Autodesk Inventor part; units mm, degrees
ref_plane "YZ Plane" through (0, 0, 0) normal (1, 0, 0) x (0, 1, 0)
ref_plane "XZ Plane" through (0, 0, 0) normal (0, 1, 0) x (-1, 0, 0)
ref_plane "XY Plane" through (0, 0, 0) normal (0, 0, 1) x (1, 0, 0)
sketch "Skizze1" plane through (0, 0, 0) normal (0, 0, 1) x (1, 0, 0)
  line L0 (-2.05, 0.55) -> (2.05, 0.55)
  line L1 (2.05, 0.55) -> (2.05, -0.55)
  line L2 (2.05, -0.55) -> (-2.05, -0.55)
  line L3 (-2.05, -0.55) -> (-2.05, 0.55)
  line L4 (-0.65, 2.05) -> (0.65, 2.05)
  line L5 (0.65, 2.05) -> (0.65, -2.05)
  line L6 (0.65, -2.05) -> (-0.65, -2.05)
  line L7 (-0.65, -2.05) -> (-0.65, 2.05)
  circle A0 centre (0, 0) radius 3.5
  line L8 (-4.9, 0) -> (4.9, 0) construction
  line L9 (0, -4.9) -> (0, 4.9) construction
  point P0 (0.65, -0.55)
  point P1 (-0.65, -0.55)
  point P2 (-0.65, 0.55)
  point P3 (0.65, 0.55)
  dimension "d0" = 1.3
  dimension "d1" = 1.1
  dimension "d2" = 4.1
  dimension "d3" = 4.1
  dimension "d4" = 7
extrude "Extrusion1" add sketch "Skizze1" along normal blind 5
sketch "Skizze2" plane through (0, 0, 5) normal (0, 0, 1) x (1, 0, 0)
  circle A0 centre (0, 0) radius 3.5
extrude "Extrusion2" add sketch "Skizze2" along normal blind 5
sketch "Skizze3" plane through (0, 0, 10) normal (0, 0, 1) x (1, 0, 0)
  circle A0 centre (0, 0) radius 6
  dimension "d9" = 12
extrude "Extrusion3" add sketch "Skizze3" along normal blind 4
chamfer "Fase1" distance 0.3 angle 60 1 edges at (-6, 0, 14) measured on face at (-0.7092, 1.4219, 14)
fillet "Rundung1" radius 0.3 1 edges at (-3.5, 0, 10)
chamfer "Fase2" distance 0.2 angle 45 1 edges at (-3.5, 0, 0)
fillet "Rundung2" radius 0.3 4 edges at (0.65, -0.55, 2.5) (-0.65, -0.55, 2.5) (0.65, 0.55, 2.5) (-0.65, 0.55, 2.5)
properties part number "Totmannknopf"
Verification items for the finished model (mm, model axes). A direction names the side the tool comes from. Coordinates: 2 decimals unless noted, no trailing zeros. Loops run counter-clockwise (first coordinate to the right, second up) from the corner with the lowest first, then second, coordinate; pieces in that order, holes last. Notation, with made-up numbers: (50.25, 73) -> (88.25, 73) arc R24 ccw to (88.25, 94) -> close; hole circle Ø10 at (73, 29). An arc over 180 degrees is marked (long way). Answer in a Markdown table with one row per item. Add a question column.
1. Depth check by flat-ended pin: P1, Ø1.5, axis at y = -3.5, z = 11, coming from the -X side; P2, Ø0.6, axis at x = 0, z = 2, coming from the +Y side; P3, Ø1, axis at x = 1.5, z = 7, coming from the -Y side. Enter the tip coordinate at first touch or a pass-through.
2. Draft check along Y on faces 3 (the face through (0, 0, 14)), 4 (the face through (2.05, 0, 2)), 5 (the face through (-6, 0, 12)). Enter one of: +Y half, -Y half, draft (parallel to the pull), parting line (faces both ways), or undercut.
3. Section check D-D, the plane z = 13. Enter the section's corners in (x, y), then the cut area to 3 significant figures.
4. Access from +Z, -Z, +X, -X, +Y, -Y to the whole of each face (thin tool, end or side, straight path). Record for faces 1 (the face through (-1, -1, 0)), 2 (the face through (-1.5, 0.55, 2.5)).
5. Section check C-C, the plane z = 3.5. Enter the section's corners in (x, y).
6. Material ranges on probe 1 along Z at (x, y) = (-0.75, 4.75); probe 2 along Z at (x, y) = (-1.5, 0.5); probe 3 along X at (y, z) = (0.5, 2), recorded low to high. Write a range as [from, to].
7. Section check A-A, the plane x = 0. Enter the section's corners in (y, z).
Derived:
| question | item | result |
|---|---|---|
| 1 | P1 | stops at x = -5.33 |
| 1 | P2 | stops at y = 3.5 |
| 1 | P3 | stops at y = -3.35 |
| 2 | face 3 | draft |
| 2 | face 4 | undercut |
| 2 | face 5 | parting line |
| 3 | outline | circle Ø12 at (0, 0) |
| 3 | area | 113 mm² |
| 4 | face 1 | -Z, +X, -X, +Y, -Y |
| 4 | face 2 | -Z |
| 5 | outline | circle Ø7 at (0, 0); hole (-2.05, -0.55) -> (-0.95, -0.55) arc R0.3 cw to (-0.65, -0.85) -> (-0.65, -2.05) -> (0.65, -2.05) -> (0.65, -0.85) arc R0.3 cw to (0.95, -0.55) -> (2.05, -0.55) -> (2.05, 0.55) -> (0.95, 0.55) arc R0.3 cw to (0.65, 0.85) -> (0.65, 2.05) -> (-0.65, 2.05) -> (-0.65, 0.85) arc R0.3 cw to (-0.95, 0.55) -> (-2.05, 0.55) -> close |
| 6 | probe 1 | z = [10, 14] |
| 6 | probe 2 | z = [5, 14] |
| 6 | probe 3 | x = [-3.46, -2.05], [2.05, 3.46] |
| 7 | outline | (-6, 10) -> (-3.8, 10) arc R0.3 cw to (-3.5, 9.7) -> (-3.5, 0.2) -> (-3.3, 0) -> (-2.05, 0) -> (-2.05, 5) -> (2.05, 5) -> (2.05, 0) -> (3.3, 0) -> (3.5, 0.2) -> (3.5, 9.7) arc R0.3 cw to (3.8, 10) -> (6, 10) -> (6, 13.48) -> (5.7, 14) -> (-5.7, 14) -> (-6, 13.48) -> close |
